```python
from build123d import *

# Parameters (mm, degrees)
SKETCH_1_W          = 240
SKETCH_1_H          = 166
EXTRUDE_1272_DEPTH  = 3
SKETCH_4_R          = 2.1
SKETCH_4_R_2        = 1.55
CUT_EXTRUDE_3_DEPTH = 251.068459046
SKETCH_5_R          = 1.55
SKETCH_5_R_2        = 10
SKETCH_5_W          = 79
SKETCH_5_H          = 45
CUT_EXTRUDE_4_DEPTH = 251.068459046
SKETCH_6_W          = 75
SKETCH_6_H          = 110
SKETCH_6_R          = 2.1
EXTRUDE_1_DEPTH     = 3
FILLET_1_R          = 5
SKETCH_8_R          = 39
CUT_EXTRUDE_6_DEPTH = 10
CUT_EXTRUDE_START   = -10
SKETCH_9_R          = 1.55
SKETCH_9_R_2        = 1.6
CUT_EXTRUDE_7_DEPTH = 10
SKETCH_10_W         = 250
SKETCH_10_H         = 82
CUT_EXTRUDE_8_DEPTH = 10


with BuildPart() as part:
    # 草图1 → Extrude 1272 (new body)
    with BuildSketch(Plane(origin=(0, 0, 0), x_dir=(1, 0, 0), z_dir=(0, 1, 0))):
        with Locations((31.575924772, -115.871750732)):
            Rectangle(SKETCH_1_W, SKETCH_1_H)
    extrude(amount=EXTRUDE_1272_DEPTH)

    # 草图4 → 切除-拉伸3 (cut, through all)
    with BuildSketch(Plane(origin=(0, 3, 0), x_dir=(1, 0, 0), z_dir=(0, 1, 0))):
        with Locations(Location((-73.424075228, -73.871750732, 0), (0, 0, 270))):
            Circle(SKETCH_4_R)
        with Locations(Location((136.575924772, -178.871750732, 0), (0, 0, 90))):
            Circle(SKETCH_4_R)
        with Locations(Location((-73.424075228, -108.871750732, 0), (0, 0, 270))):
            Circle(SKETCH_4_R)
        with Locations(Location((-73.424075228, -143.871750732, 0), (0, 0, 270))):
            Circle(SKETCH_4_R)
        with Locations(Location((-73.424075228, -178.871750732, 0), (0, 0, 270))):
            Circle(SKETCH_4_R)
        with Locations(Location((136.575924772, -143.871750732, 0), (0, 0, 90))):
            Circle(SKETCH_4_R)
        with Locations(Location((136.575924772, -108.871750732, 0), (0, 0, 90))):
            Circle(SKETCH_4_R)
        with Locations(Location((136.575924772, -73.871750732, 0), (0, 0, 90))):
            Circle(SKETCH_4_R)
        with Locations(Location((-73.424075228, -38.871750732, 0), (0, 0, 270))):
            Circle(SKETCH_4_R)
        with Locations(Location((136.575924772, -38.871750732, 0), (0, 0, 90))):
            Circle(SKETCH_4_R)
        with Locations(Location((77.075924772, -188.871750732, 0), (0, 0, 270))):
            Circle(SKETCH_4_R_2)
        with Locations(Location((-13.924075228, -188.871750732, 0), (0, 0, 90))):
            Circle(SKETCH_4_R_2)
        with Locations(Location((77.075924772, -153.871750732, 0), (0, 0, 270))):
            Circle(SKETCH_4_R_2)
        with Locations(Location((-13.924075228, -153.871750732, 0), (0, 0, 90))):
            Circle(SKETCH_4_R_2)
    extrude(amount=-CUT_EXTRUDE_3_DEPTH, mode=Mode.SUBTRACT)

    # 草图5 → 切除-拉伸4 (cut, through all)
    with BuildSketch(Plane(origin=(0, 3, 0), x_dir=(1, 0, 0), z_dir=(0, 1, 0))):
        with Locations(Location((-5.424075228, -51.871750732, 0), (0, 0, 270))):
            Circle(SKETCH_5_R)
        with Locations(Location((68.575924772, -51.871750732, 0), (0, 0, 90))):
            Circle(SKETCH_5_R)
        with Locations(Location((68.575924772, -108.871750732, 0), (0, 0, 270))):
            Circle(SKETCH_5_R)
        with Locations(Location((-5.424075228, -108.871750732, 0), (0, 0, 90))):
            Circle(SKETCH_5_R)
        with Locations(Location((-45.424075228, -143.871750732, 0), (0, 0, 270))):
            Circle(SKETCH_5_R_2)
        with Locations(Location((108.575924772, -143.871750732, 0), (0, 0, 90))):
            Circle(SKETCH_5_R_2)
        with Locations((31.575924772, -80.371750732)):
            Rectangle(SKETCH_5_W, SKETCH_5_H)
        with BuildLine():
            Line((86.075924772, -100.371750732), (86.075924772, -60.371750732))
            ThreePointArc((86.075924772, -60.371750732), (91.075924772, -55.371750732), (96.075924772, -60.371750732))
            Line((96.075924772, -60.371750732), (96.075924772, -100.371750732))
            ThreePointArc((96.075924772, -100.371750732), (91.075924772, -105.371750732), (86.075924772, -100.371750732))
        make_face()
        with BuildLine():
            Line((1.575924772, -117.871750732), (61.575924772, -117.871750732))
            ThreePointArc((61.575924772, -117.871750732), (68.575924772, -124.871750732), (61.575924772, -131.871750732))
            Line((61.575924772, -131.871750732), (41.575924772, -131.871750732))
            ThreePointArc((41.575924772, -131.871750732), (31.575924772, -141.871750732), (21.575924772, -131.871750732))
            Line((21.575924772, -131.871750732), (1.575924772, -131.871750732))
            ThreePointArc((1.575924772, -131.871750732), (-5.424075228, -124.871750732), (1.575924772, -117.871750732))
        make_face()
    extrude(amount=-CUT_EXTRUDE_4_DEPTH, mode=Mode.SUBTRACT)

    # 草图6 → 凸台-拉伸1 (add)
    # profile 1 of 2: a face of its own
    with BuildSketch(Plane(origin=(0, 0, 0), x_dir=(1, 0, 0), z_dir=(0, 1, 0))):
        with Locations((-125.924075228, -108.871750732)):
            Rectangle(SKETCH_6_W, SKETCH_6_H)
        with Locations(Location((-153.424075228, -61.371750732, 0), (0, 0, 270))):
            Circle(SKETCH_6_R, mode=Mode.SUBTRACT)
        with Locations(Location((-153.424075228, -156.371750732, 0), (0, 0, 90))):
            Circle(SKETCH_6_R, mode=Mode.SUBTRACT)
        with Locations(Location((-128.424075228, -61.371750732, 0), (0, 0, 270))):
            Circle(SKETCH_6_R, mode=Mode.SUBTRACT)
        with Locations(Location((-128.424075228, -156.371750732, 0), (0, 0, 90))):
            Circle(SKETCH_6_R, mode=Mode.SUBTRACT)
    # profile 2 of 2: a face of its own
    with BuildSketch(Plane(origin=(0, 0, 0), x_dir=(1, 0, 0), z_dir=(0, 1, 0))):
        with Locations((189.075924772, -108.871750732)):
            Rectangle(SKETCH_6_W, SKETCH_6_H)
        with Locations(Location((216.575924772, -156.371750732, 0), (0, 0, 270))):
            Circle(SKETCH_6_R, mode=Mode.SUBTRACT)
        with Locations(Location((216.575924772, -61.371750732, 0), (0, 0, 90))):
            Circle(SKETCH_6_R, mode=Mode.SUBTRACT)
        with Locations(Location((191.575924772, -156.371750732, 0), (0, 0, 270))):
            Circle(SKETCH_6_R, mode=Mode.SUBTRACT)
        with Locations(Location((191.575924772, -61.371750732, 0), (0, 0, 90))):
            Circle(SKETCH_6_R, mode=Mode.SUBTRACT)
    extrude(amount=EXTRUDE_1_DEPTH)

    # 圆角1
    fillet_1_edges = [part.edges().sort_by_distance(p)[0] for p in [
        (41.575924772, 1.5, 131.871750732),
        (21.575924772, 1.5, 131.871750732),
        (-7.924075228, 1.5, 102.871750732),
        (-7.924075228, 1.5, 57.871750732),
        (71.075924772, 1.5, 57.871750732),
        (71.075924772, 1.5, 102.871750732),
        (-88.424075228, 1.5, 163.871750732),
        (-88.424075228, 1.5, 53.871750732),
        (-163.424075228, 1.5, 53.871750732),
        (-163.424075228, 1.5, 163.871750732),
        (226.575924772, 1.5, 53.871750732),
        (151.575924772, 1.5, 53.871750732),
        (151.575924772, 1.5, 163.871750732),
        (226.575924772, 1.5, 163.871750732),
        (-88.424075228, 1.5, 198.871750732),
        (-88.424075228, 1.5, 32.871750732),
        (151.575924772, 1.5, 32.871750732),
        (151.575924772, 1.5, 198.871750732),
    ]]
    fillet(fillet_1_edges, radius=FILLET_1_R)

    # 草图8 → 切除-拉伸6 (cut)
    with BuildSketch(Plane(origin=(0, 3, 0), x_dir=(1, 0, 0), z_dir=(0, 1, 0))):
        with Locations((31.575924772, -158.205226673)):
            Circle(SKETCH_8_R)
    extrude(amount=-CUT_EXTRUDE_6_DEPTH, mode=Mode.SUBTRACT)

    # 草图9 → 切除-拉伸7 (cut)
    with BuildSketch(Plane.XZ.offset(CUT_EXTRUDE_START)):
        with Locations(Location((68.575924772, 108.871750732, 0), (0, 0, 90))):
            Circle(SKETCH_9_R)
        with Locations(Location((-48.424075228, 108.871750732, 0), (0, 0, 270))):
            Circle(SKETCH_9_R)
        with Locations(Location((25.575924772, 108.871750732, 0), (0, 0, 270))):
            Circle(SKETCH_9_R)
        with Locations(Location((25.575924772, 51.871750732, 0), (0, 0, 90))):
            Circle(SKETCH_9_R)
        with Locations(Location((-48.424075228, 51.871750732, 0), (0, 0, 90))):
            Circle(SKETCH_9_R)
        with Locations(Location((114.075924772, 51.871750732, 0), (0, 0, 270))):
            Circle(SKETCH_9_R)
        with Locations(Location((114.075924772, 74.371750732, 0), (0, 0, 270))):
            Circle(SKETCH_9_R_2)
        with Locations(Location((114.075924772, 86.371750732, 0), (0, 0, 90))):
            Circle(SKETCH_9_R_2)
        with Locations(Location((114.075924772, 108.871750732, 0), (0, 0, 90))):
            Circle(SKETCH_9_R)
        with Locations(Location((114.075924772, 131.371750732, 0), (0, 0, 270))):
            Circle(SKETCH_9_R_2)
        with Locations(Location((68.075924772, 131.371750732, 0), (0, 0, 90))):
            Circle(SKETCH_9_R_2)
    extrude(amount=CUT_EXTRUDE_7_DEPTH, mode=Mode.SUBTRACT)

    # 草图10 → 切除-拉伸8 (cut)
    with BuildSketch(Plane.XZ):
        with Locations((31.575924772, 157.871750732)):
            Rectangle(SKETCH_10_W, SKETCH_10_H)
    extrude(amount=-CUT_EXTRUDE_8_DEPTH, mode=Mode.SUBTRACT)


solid = part.part
```
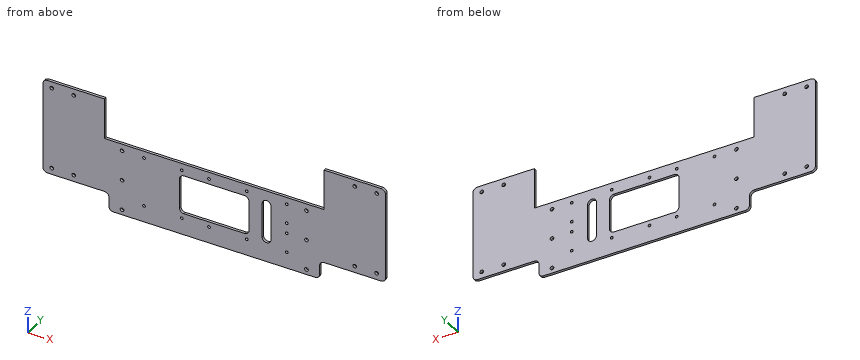
Input: part model. Units: mm. Frame: model coordinates. Round coordinates to 2 decimals unless told otherwise and drop trailing zeros. Write each loop counter-clockwise with the first axis right and the second up, starting at its lowest first coordinate (ties: lowest second). Pieces come first, ordered by that corner, then holes. Notation, with made-up numbers: (-25, -24.75) - (-14, -24.75) arc R19 cw to (-14, -3.75) - close; hole circle Ø10 at (76.25, -23.5). An arc over 180 degrees is marked (long way). Write item = value, one per line.
(1) Section query A-A on z = 140.5. Output: boundary loops of the cut face in (x, y), then the cut area to 3 significant figures.
Geometry check:
outline = (-163.42, 0) - (-93.42, 0) - (-93.42, 3) - (-163.42, 3) - close; (156.58, 0) - (226.58, 0) - (226.58, 3) - (156.58, 3) - close
area = 420 mm^2
(2) Material intervals for probe 1 along X at (y, z) = (1.45, 81); probe 2 along Z at (x, y) = (50, 1.5); probe 3 along X at (y, z) = (1.1, 140.5), sorted ascending.
Geometry check:
probe_1 = -163.42 to -7.92, 71.08 to 86.08, 96.08 to 226.58
probe_2 = 32.87 to 57.87, 102.87 to 116.87
probe_3 = -163.42 to -93.42, 156.58 to 226.58
(3) Section query D-D on x = 76. Output: boundary loops of the cut face in (y, z), then the cut area to 3 significant figures.
Geometry check:
outline = (0, 32.87) - (3, 32.87) - (3, 116.87) - (0, 116.87) - close
area = 252 mm^2
(4) Section query C-C on y = 0.6. State how many separate pieces and enclosed holes the cut face has, then the cut area to 3 significant figures.
Geometry check:
separate_pieces = 1
enclosed_holes = 28
area = 31,900 mm^2
(5) Section query B-B on x = -120.5. Output: boundary loops of the cut face in (y, z).
Geometry check:
outline = (0, 53.87) - (3, 53.87) - (3, 163.87) - (0, 163.87) - close
(6) Contact query for flat-ended pins moving along their axis: pin 1 Ø4 at (x, z) = (-73.42, 73.87) entering from +Y (3 decimals); pin 2 Ø4 at (x, z) = (68.58, 51.87) entering from +Y; pin 3 Ø1 at (x, y) = (38.5, 1.5) entering from +Z; pin 4 Ø1 at (x, y) = (172, 2.5) entering from -Z. Output: stop coordinate, or through.
Geometry check:
pin_1 = through
pin_2 = 3
pin_3 = 116.87
pin_4 = 53.87
